Input: dimensioned drawing with shaded views. Units: mm. Origin: part minimum x, y, z. Coordinates: 2 decimals unless noted, no trailing zeros. Loops run counter-clockwise (first coordinate to the right, second up) from the corner with the lowest first, then second, coordinate; pieces in that order, holes last. Notation, with made-up numbers: (17.25, -34.5) - (31.25, -34.5) arc R10 ccw to (31.25, -22.5) - close; hole circle Ø4 at (-27, -27). An arc over 180 degrees is marked (long way). Put each result on its own line as item: value. Start each with the question number.
1) Section B-B on z = 79.5. Output: boundary loops of the cut face in (x, y).
2) Section A-A on x = 28. Output: boundary loops of the cut face in (y, z), and give its area (3 significant figures).
3) Section C-C on x = 99.75. Output: boundary loops of the cut face in (y, z), and give its area (3 significant figures).
4) Material intervals for line 1 along X through (y, z) = (2.2, 40.5); line 2 along Z through (x, y) = (62, 0.4); line 3 along X through (y, z) = (0.3, 90.5), sorted ascending. Write a range as from..to.
5) Section D-D on z = 55.5. Output: boundary loops of the cut face in (x, y).
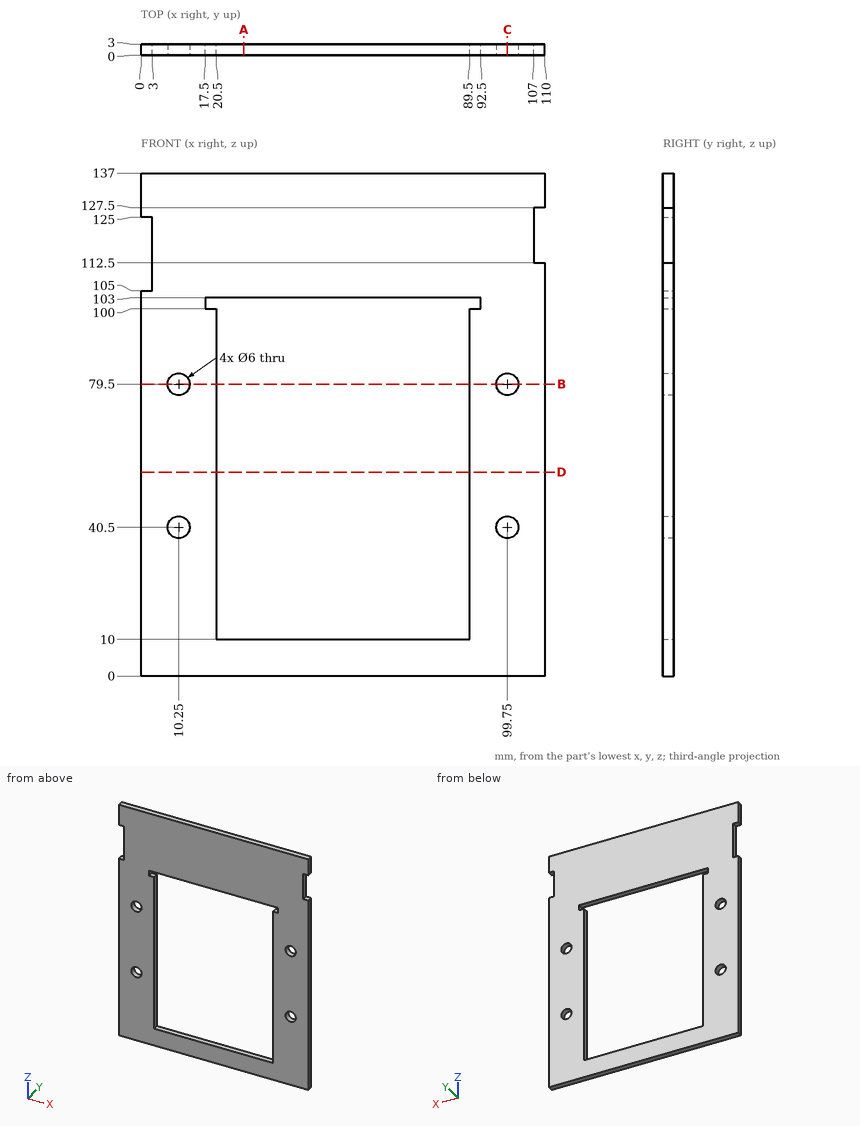
Answer block:
1. outline: (0, 0) - (7.25, 0) - (7.25, 3) - (0, 3) - close; (13.25, 0) - (20.5, 0) - (20.5, 3) - (13.25, 3) - close; (89.5, 0) - (96.75, 0) - (96.75, 3) - (89.5, 3) - close; (102.75, 0) - (110, 0) - (110, 3) - (102.75, 3) - close
2. outline: (0, 0) - (3, 0) - (3, 10) - (0, 10) - close; (0, 103) - (3, 103) - (3, 137) - (0, 137) - close
2. area: 132 mm²
3. outline: (0, 0) - (3, 0) - (3, 37.5) - (0, 37.5) - close; (0, 43.5) - (3, 43.5) - (3, 76.5) - (0, 76.5) - close; (0, 82.5) - (3, 82.5) - (3, 137) - (0, 137) - close
3. area: 375 mm²
4. line 1: x = 0..7.25, 13.25..20.5, 89.5..96.75, 102.75..110
4. line 2: z = 0..10, 103..137
4. line 3: x = 0..20.5, 89.5..110
5. outline: (0, 0) - (20.5, 0) - (20.5, 3) - (0, 3) - close; (89.5, 0) - (110, 0) - (110, 3) - (89.5, 3) - close
